from build123d import *

# Parameters (mm, degrees)
BOSS_EXTRUDE1_DEPTH = 20
SKETCH2_R           = 3
CUT_EXTRUDE1_DEPTH  = 4
SKETCH3_R           = 3
CUT_EXTRUDE2_DEPTH  = 4
FILLET1_R           = 5
SKETCH4_W           = 20
SKETCH4_H           = 4
BOSS_EXTRUDE2_DEPTH = 10
SKETCH5_W           = 20
SKETCH5_H           = 4
BOSS_EXTRUDE3_DEPTH = 10
SKETCH6_R           = 1.5
CUT_EXTRUDE3_DEPTH  = 4


with BuildPart() as part:
    # Sketch1 → Boss-Extrude1 (new body)
    with BuildSketch(Plane.XY):
        Polygon((-89.731830747, 25.752777778), (-89.731830747, -4.247222222), (10.268169253, -4.247222222), (10.268169253, 25.752777778), (14.268169253, 25.752777778), (14.268169253, -8.247222222), (-93.731830747, -8.247222222), (-93.731830747, 25.752777778), align=None)
    extrude(amount=BOSS_EXTRUDE1_DEPTH)

    # Sketch2 → Cut-Extrude1 (cut)
    with BuildSketch(Plane.ZY.offset(93.731830747)):
        with Locations((10, 10.752777778)):
            Circle(SKETCH2_R)
    extrude(amount=-CUT_EXTRUDE1_DEPTH, mode=Mode.SUBTRACT)

    # Sketch3 → Cut-Extrude2 (cut)
    with BuildSketch(Plane(origin=(14.268169253, 0, 0), x_dir=(0, 0, -1), z_dir=(1, 0, 0))):
        with Locations((-10, 10.752777778)):
            Circle(SKETCH3_R)
    extrude(amount=-CUT_EXTRUDE2_DEPTH, mode=Mode.SUBTRACT)

    # Fillet1
    fillet1_edges = [part.edges().sort_by_distance(p)[0] for p in [
        (-91.731830747, 25.752777778, 0),
        (12.268169253, 25.752777778, 20),
        (-91.731830747, 25.752777778, 20),
        (12.268169253, 25.752777778, 0),
    ]]
    fillet(fillet1_edges, radius=FILLET1_R)

    # Sketch4 → Boss-Extrude2 (add)
    with BuildSketch(Plane(origin=(14.268169253, 0, 0), x_dir=(0, 0, -1), z_dir=(1, 0, 0))):
        with Locations((-10, -6.247222222)):
            Rectangle(SKETCH4_W, SKETCH4_H)
    extrude(amount=BOSS_EXTRUDE2_DEPTH)

    # Sketch5 → Boss-Extrude3 (add)
    with BuildSketch(Plane.ZY.offset(93.731830747)):
        with Locations((10, -6.247222222)):
            Rectangle(SKETCH5_W, SKETCH5_H)
    extrude(amount=BOSS_EXTRUDE3_DEPTH)

    # Sketch6 → Cut-Extrude3 (cut)
    with BuildSketch(Plane(origin=(0, -4.247222222, 0), x_dir=(1, 0, 0), z_dir=(0, 1, 0))):
        with Locations((-98.731830747, -10)):
            Circle(SKETCH6_R)
        with Locations((19.268169253, -10)):
            Circle(SKETCH6_R)
    extrude(amount=-CUT_EXTRUDE3_DEPTH, mode=Mode.SUBTRACT)


solid = part.part
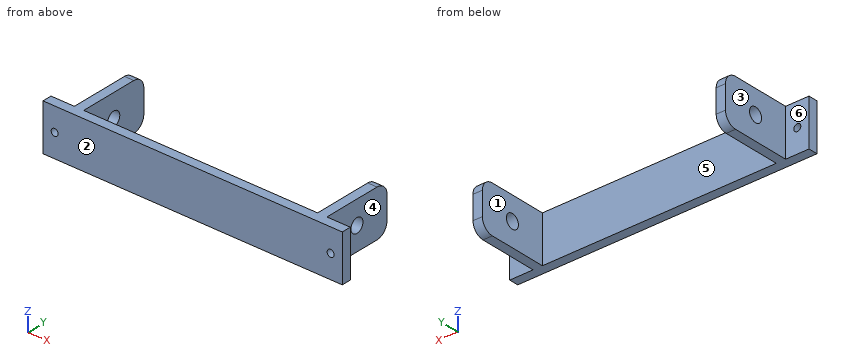
CAD build for the part. Positions are in the model's coordinates, mm. Face numbers are marked on the shaded views. A direction names the side the tool comes from. Give positions to 0.01 mm unless a question says otherwise; leave off trailing zeros. Loops run counter-clockwise (first coordinate to the right, second up) from the corner with the lowest first, then second, coordinate; pieces in that order, holes last. Notation, with made-up numbers: M 3,19 L 27,19 A6 cw 27,27 Z; hole C 10,13.25 d1. An arc over 180 degrees is marked long. One line per question, with ' | ' between items. Start each with the question number.
1. Saw through at A-A on z = 10. Give the cut face in (x, y).
2. Probe L1, parallel to X at y = -7.2, z = 10; L2, parallel to X at y = 2, z = 14; L3, parallel to Y at x = 13.1, z = 10. List the from-to ranges inside material, lowest first. Write a range as from..to.
3. Saw through at C-C on x = 13. Give the cut face in (y, z).
4. Flat gauge pins, fed straight in: pin 1 (10 mm diameter, centred on y = 18, z = 8, fed in from +X); pin 2 (3 mm diameter, centred on x = 21, z = 13.5, fed in from +Y); pin 3 (10 mm diameter, centred on y = 6.5, z = 9, fed in from -X). Where does each tip first touch, or does it go through?
5. Saw through at B-B on y = 4.5. Give the cut face in (x, z).
6. 3-axis set-ups, long thin cutter, end or side, ignore diameter. For the marked faces 1, 2 and 3: which of +Z, -Z, +X, -X, +Y, -Y reach the whole face in a straight line?
7. Two-plate mould, pull along X, no slides. Class the marked faces 4, 5 and 6: pulls with the +X half, pulls with the -X half, needs draft (parallel to the pull), parting line crosses it, or undercut.
8. Saw through at D-D on x = -59.5. Give the cut face in (y, z).
Result sheet:
1) outline: M -103.73,-8.25 L -100.23,-8.25 L -100.23,-4.25 L -103.73,-4.25 Z; M -97.23,-8.25 L 17.77,-8.25 L 17.77,-4.25 L 14.27,-4.25 L 14.27,7.75 L 10.27,7.75 L 10.27,-4.25 L -89.73,-4.25 L -89.73,7.75 L -93.73,7.75 L -93.73,-4.25 L -97.23,-4.25 Z; M -93.73,13.75 L -89.73,13.75 L -89.73,25.75 L -93.73,25.75 Z; M 10.27,13.75 L 14.27,13.75 L 14.27,25.75 L 10.27,25.75 Z; M 20.77,-8.25 L 24.27,-8.25 L 24.27,-4.25 L 20.77,-4.25 Z
2) L1: x = -103.73..-100.23, -97.23..17.77, 20.77..24.27 | L2: x = -93.73..-89.73, 10.27..14.27 | L3: y = -8.25..7.75, 13.75..25.75
3) outline: M -8.25,0 L 20.75,0 A5 ccw 25.75,5 L 25.75,15 A5 ccw 20.75,20 L -8.25,20 Z; hole C 10.75,10 d6
4) pin 1: stops at x = 14.27 | pin 2: stops at y = -4.25 | pin 3: stops at x = -93.73
5) outline: M -93.73,0 L -89.73,0 L -89.73,20 L -93.73,20 Z; M 10.27,0 L 14.27,0 L 14.27,20 L 10.27,20 Z
6) face 1: +Z, -Z, +Y | face 2: +Z, -Z, +X, -X, -Y | face 3: +Z, -Z, -X, +Y
7) face 4: pulls with the +X half | face 5: undercut | face 6: needs draft
8) outline: M -8.25,0 L -4.25,0 L -4.25,20 L -8.25,20 Z
